Geometry: final body of the model. Coordinates: model frame, mm. A direction names the side the tool comes from. Coordinates: 2 decimals unless noted, no trailing zeros. Write each loop counter-clockwise with the first axis right and the second up, starting at its lowest first coordinate (ties: lowest second). Pieces come first, ordered by that corner, then holes. Notation, with made-up numbers: (-37.5, 6.5) -> (10.5, 6.5) arc R18 cw to (10.5, 35.5) -> close; hole circle Ø5 at (-19.75, 89). An arc over 180 degrees is marked (long way). One line per item, written item: value. Start each with the question number.
Autodesk Inventor part; units mm, degrees
ref_plane "YZ Plane" through (0, 0, 0) normal (1, 0, 0) x (0, 1, 0)
ref_plane "XZ Plane" through (0, 0, 0) normal (0, 1, 0) x (-1, 0, 0)
ref_plane "XY Plane" through (0, 0, 0) normal (0, 0, 1) x (1, 0, 0)
sketch "Sketch1" plane through (0, 0, 0) normal (0, 1, 0) x (-1, 0, 0)
  circle A0 centre (0, 0) radius 2.25
  line L0 (-2, 5) -> (2, 5)
  line L1 (5, 2) -> (5, -31.75)
  line L2 (5, -31.75) -> (-5, -31.75)
  line L3 (-5, -31.75) -> (-5, 2)
  line L4 (-5, -28.75) -> (5, -28.75)
  arc A1 (-2, 5) -> (-5, 2) centre (-2, 2) ccw
  arc A2 (5, 2) -> (2, 5) centre (2, 2) ccw
  point P0 (-5, 5)
  point P1 (5, 5)
  dimension "d0" = 4.5
  dimension "d3" = 5
  dimension "d4" = 10
  dimension "d5" = 36.75
  dimension "d6" = 3
  dimension "d9" = 3
extrude "Extrusion1" add sketch "Sketch1" along normal blind 3
extrude "Extrusion2" add sketch "Sketch1" along normal blind 13 contours L4 L1 L2 L3
sketch "Sketch2" plane through (-5, 3, -28.75) normal (0, 0, 1) x (1, 0, 0)
  circle A0 centre (5, 5) radius 2.25
  circle A1 centre (5, 5) radius 4.25
  point P0 (5, -3)
  dimension "d12" = 4.5
  dimension "d16" = 2
extrude "Extrusion3" cut sketch "Sketch2" against normal blind 4 contours A0
fillet "Fillet1" radius 5 1 edges at (0, 3, -28.75)
extrude "Extrusion4" cut sketch "Sketch2" along normal blind 4
properties part number "GearStand"
Q1. Line query: L1, parallel to X at y = 8, z = -30.6; L2, parallel to Y at x = 0, z = -30.05; L3, parallel to Z at x = 0, y = 1.35. Output: solid intervals per line, ascending. Write a range as from..to.
Q2. First-contact query: P1, Ø2.5, axis at x = 0, z = 0, coming from the +Y side; P2, Ø1, axis at x = -2, z = -20, coming from the +Y side. Flat tips, straight axial feed; report the tip coordinate or a pass-through.
Q3. Cut plane B-B on y = 2.25. Output: boundary loops of the cut face in (x, z), and give its area (3 significant figures).
Q4. Cut plane C-C on z = 0. Output: boundary loops of the cut face in (x, y), and give its area (3 significant figures).
Q5. Draft query along X for faces 1 (the cylindrical face through (0.09, 3.75, -27.85)), 2 (the flat face through (0, 0, -13)), 3 (the flat face through (5, 2.6, -18.7)). Return one class per face: pulls with the +X half, pulls with the -X half, needs draft (parallel to the pull), parting line crosses it, or undercut.
Q6. Cut plane D-D on y = 6.5. Output: boundary loops of the cut face in (x, z), and give its area (3 significant figures).
Q7. Access query for faces 4 (the flat face through (0.1, 10.4, -28.75)), 5 (the flat face through (-5, 2, -19)), 6 (the flat face through (0, 3, -9)). Directions: +Z, -Z, +X, -X, +Y, -Y. A direction counts if a zero-diameter tool reaches every point of the face in a straight line with its end or side. Return the directions, or none.
Q8. Cut plane A-A on x = 0. Output: boundary loops of the cut face in (y, z).
Solution:
1. L1: -5..-2.25, 2.25..5
1. L2: 0..5.75, 10.25..13
1. L3: -31.75..-2.25, 2.25..5
2. P1: through
2. P2: y = 3
3. outline: (-5, -31.75) -> (5, -31.75) -> (5, 2) arc R3 ccw to (2, 5) -> (-2, 5) arc R3 ccw to (-5, 2) -> close; hole circle Ø4.5 at (0, 0)
3. area: 348 mm²
4. outline: (-5, 0) -> (-2.25, 0) -> (-2.25, 3) -> (-5, 3) -> close; (2.25, 0) -> (5, 0) -> (5, 3) -> (2.25, 3) -> close
4. area: 16.5 mm²
5. face 1: undercut
5. face 2: needs draft
5. face 3: pulls with the +X half
6. outline: (-5, -31.75) -> (-1.68, -31.75) -> (-1.68, -28.75) -> (-3.98, -28.75) -> (-3.98, -28.52) -> (-5, -28.52) -> close; (1.68, -31.75) -> (5, -31.75) -> (5, -28.52) -> (3.98, -28.52) -> (3.98, -28.75) -> (1.68, -28.75) -> close
6. area: 20.4 mm²
7. face 4: +Z, +Y
7. face 5: +Z, -Z, -X, +Y, -Y
7. face 6: +Z, +X, -X, +Y
8. outline: (0, -31.75) -> (5.75, -31.75) -> (5.75, -28.75) -> (3.75, -28.75) -> (3.75, -26.38) arc R5 cw to (3, -23.75) -> (3, -2.25) -> (0, -2.25) -> close; (0, 2.25) -> (3, 2.25) -> (3, 5) -> (0, 5) -> close; (10.25, -31.75) -> (13, -31.75) -> (13, -28.75) -> (10.25, -28.75) -> close
